Design review of the part built by this model. Coordinates are the model's own, in mm. Coordinates: 2 decimals unless noted, no trailing zeros. Write each loop counter-clockwise with the first axis right and the second up, starting at its lowest first coordinate (ties: lowest second). Pieces come first, ordered by that corner, then holes. Notation, with made-up numbers: (35.25, 39.5) -> (90.25, 39.5) arc R26 ccw to (90.25, 56.5) -> close; hole circle Ø4 at (-36, -1). An arc over 180 degrees is marked (long way). Answer in a Markdown table with one row per item. Add a question column.
Item 1: Take a section at B-B, the plane y = 90. Write out the cut boundary in (x, z).
Item 2: Take a section at A-A, the plane x = 0. Write out the cut boundary in (y, z), and give its area (3 significant figures).
Item 3: Take a section at C-C, the plane z = -42. Write out the cut boundary in (x, y), and give its area (3 significant figures).
Item 4: To check wall thickness, follow line 1 (X direction, y = 90, z = -42); line 2 (Y direction, x = 0, z = -45.5); line 3 (X direction, y = 92, z = -46.25). State the ranges of each line that lie inside material, in increasing order.
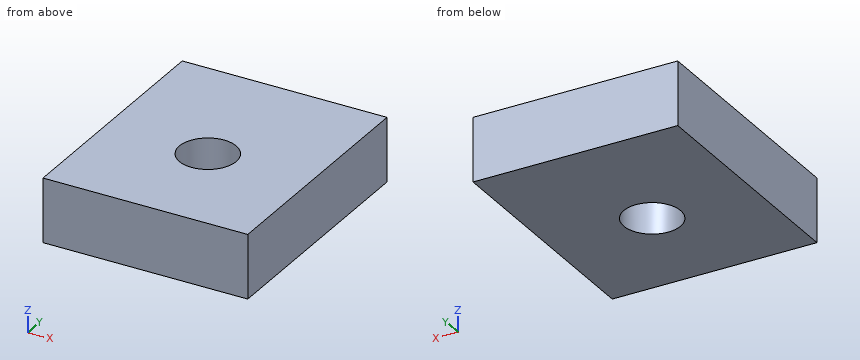
from build123d import *

# Parameters (mm, degrees)
CYLINDER1616_R     = 4
CYLINDER1616_DEPTH = 100
BOX642_W           = 28.8
BOX642_H           = 34.21
BOX642_DEPTH       = 9


with BuildPart() as obj1:
    # Cylinder1616 → Cylinder1616 (new body)
    with BuildSketch(Plane.XY):
        Circle(CYLINDER1616_R)
    extrude(amount=CYLINDER1616_DEPTH)


with BuildPart() as cut308:
    # Box642 → Box642 (new body)
    with BuildSketch(Plane(origin=(-14.4, -15.34, 34), x_dir=(1, 0, 0), z_dir=(0, 0, 1))):
        with Locations((14.4, 17.105)):
            Rectangle(BOX642_W, BOX642_H)
    extrude(amount=BOX642_DEPTH)

    # Cut308: cut obj1
    add(obj1.part, mode=Mode.SUBTRACT)


with BuildPart() as cut308_1:
    # Cut308 placement: moved
    add(cut308.part.moved(Location((0, 90, -83))))


solid = cut308_1.part
Answers:
| question | item | result |
|---|---|---|
| 1 | outline | (-14.4, -49) -> (-4, -49) -> (-4, -40) -> (-14.4, -40) -> close; (4, -49) -> (14.4, -49) -> (14.4, -40) -> (4, -40) -> close |
| 2 | outline | (74.66, -49) -> (86, -49) -> (86, -40) -> (74.66, -40) -> close; (94, -49) -> (108.87, -49) -> (108.87, -40) -> (94, -40) -> close |
| 2 | area | 236 mm^2 |
| 3 | outline | (-14.4, 74.66) -> (14.4, 74.66) -> (14.4, 108.87) -> (-14.4, 108.87) -> close; hole circle Ø8 at (0, 90) |
| 3 | area | 935 mm^2 |
| 4 | line 1 | x = -14.4 to -4, 4 to 14.4 |
| 4 | line 2 | y = 74.66 to 86, 94 to 108.87 |
| 4 | line 3 | x = -14.4 to -3.46, 3.46 to 14.4 |
